Build history of the part. All positions in model axes, mm. Round coordinates to 2 decimals unless told otherwise and drop trailing zeros. Order: outer loops, then holes, each group sorted by start corner. A loop starts at its lowest first (then second) coordinate and runs counter-clockwise, first axis right, second up. Notation, with made-up numbers: (-15, 19) -> (25, 19) arc R8 cw to (25, 27) -> close; hole circle Ø4 at (-4, -6). An arc over 180 degrees is marked (long way). Use a Markdown table: item, result. Add a question column.
Item 1: Slice it at C-C, the plane x = -10. Give the cut face in (y, z).
Item 2: Probe L1, parallel to Y at x = -20, z = 0.6 (3 decimals); L2, parallel to Y at x = -6, z = 0.5; L3, parallel to X at y = 49.5, z = 1.4. List the from-to ranges inside material, lowest first.
Item 3: Slice it at A-A, the plane z = 0.35. Give the cut face in (x, y), plus the area to 3 significant figures.
Item 4: Slice it at B-B, the plane y = 125. Give the cut face in (x, z).
Item 5: Pin check, flat tip, straight feed: pin 1 (1.5 mm diameter, centred on x = -17, y = 57.5, fed in from -Z). Stop position of the tip, or through.
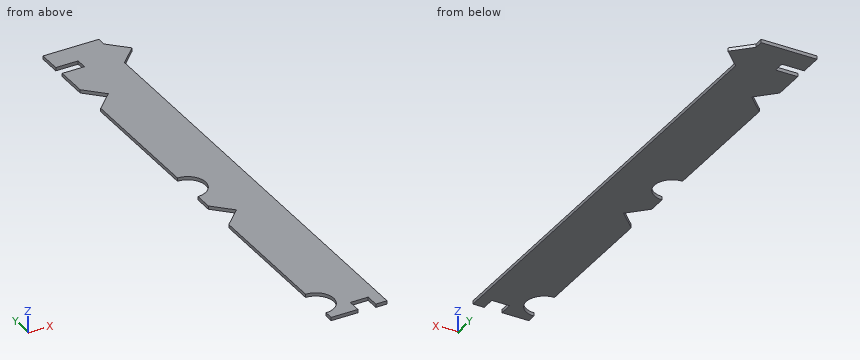
Autodesk Inventor part; units mm, degrees
ref_plane "YZ Plane" through (0, 0, 0) normal (1, 0, 0) x (0, 1, 0)
ref_plane "XZ Plane" through (0, 0, 0) normal (0, 1, 0) x (-1, 0, 0)
ref_plane "XY Plane" through (0, 0, 0) normal (0, 0, 1) x (1, 0, 0)
sketch "Sketch1" plane through (0, 0, 0) normal (0, 0, 1) x (1, 0, 0)
  circle A0 centre (0, 213.2) radius 8 construction
  line L0 (0, 221.2) -> (8, 213.2)
  line L1 (0, 205.2) -> (8, 213.2)
  line L2 (0, 0) -> (0, 205.2)
  line L3 (0, 225.2) -> (-25, 225.2)
  line L4 (-25, 0) -> (-13, 0)
  line L5 (-13, 0) -> (-13, 6)
  line L6 (-13, 6) -> (-5, 6)
  line L7 (-5, 6) -> (-5, 0)
  line L8 (-25, 0) -> (-13, 0)
  line L9 (-5, 0) -> (0, 0)
  line L10 (-25, 196.1) -> (-17, 188.1)
  line L11 (-17, 188.1) -> (-25, 180.1)
  arc A1 (-25, 104.1) -> (-25, 120.1) centre (-25, 112.1) ccw
  line L12 (-25, 180.1) -> (-25, 120.1)
  circle A2 centre (-25, 188.1) radius 8 construction
  line L13 (0, 221.2) -> (0, 225.2)
  line L14 (-25, 215.2) -> (-15, 215.2)
  line L15 (-15, 215.2) -> (-15, 210.2)
  line L16 (-15, 210.2) -> (-25, 210.2)
  line L17 (-25, 225.2) -> (-25, 215.2)
  line L18 (-25, 210.2) -> (-25, 196.1)
  arc A3 (-25, 4) -> (-25, 20) centre (-25, 12) ccw
  line L19 (-25, 4) -> (-25, 0)
  line L20 (-25, 96) -> (-17, 88)
  line L21 (-17, 88) -> (-25, 80)
  circle A4 centre (-25, 88) radius 8 construction
  line L22 (-25, 104.1) -> (-25, 96)
  line L23 (-25, 80) -> (-25, 20)
  dimension "d5" = 16
  dimension "d168" = 25
  dimension "d177" = 12
  dimension "d178" = 6
  dimension "d179" = 8
  dimension "d189" = 76
  dimension "d193" = 4
  dimension "d194" = 10
  dimension "d195" = 5
  dimension "d196" = 225.2
  dimension "d197" = 10
  dimension "d198" = 37.1
  dimension "d199" = 76
  dimension "d200" = 24.1
  dimension "d201" = 5
extrude "Extrusion10" add sketch "Sketch1" along normal blind 1.5
properties part number "MS_FI_v3"
Check sheet entries:
| question | item | result |
|---|---|---|
| 1 | outline | (6, 0) -> (225.2, 0) -> (225.2, 1.5) -> (6, 1.5) -> close |
| 2 | L1 | 0 to 5.755, 18.245 to 85, 91 to 105.855, 118.345 to 185.1, 191.1 to 210.2, 215.2 to 225.2 |
| 2 | L2 | 6 to 225.2 |
| 2 | L3 | -25 to 0 |
| 3 | outline | (-25, 0) -> (-13, 0) -> (-13, 6) -> (-5, 6) -> (-5, 0) -> (0, 0) -> (0, 205.2) -> (8, 213.2) -> (0, 221.2) -> (0, 225.2) -> (-25, 225.2) -> (-25, 215.2) -> (-15, 215.2) -> (-15, 210.2) -> (-25, 210.2) -> (-25, 196.1) -> (-17, 188.1) -> (-25, 180.1) -> (-25, 120.1) arc R8 cw to (-25, 104.1) -> (-25, 96) -> (-17, 88) -> (-25, 80) -> (-25, 20) arc R8 cw to (-25, 4) -> close |
| 3 | area | 5,270 mm2 |
| 4 | outline | (-25, 0) -> (0, 0) -> (0, 1.5) -> (-25, 1.5) -> close |
| 5 | pin 1 | z = 0 |
